For this review, take the finished solid that the model builds, in its own axes (mm). A direction names the side the tool comes from. Coordinates: 2 decimals unless noted, no trailing zeros. Loops run counter-clockwise (first coordinate to the right, second up) from the corner with the lowest first, then second, coordinate; pieces in that order, holes last.
1. Machinability: for faces 1 (the face through (32, 24, -11)), 2 (the face through (35.5, 16, -61)), 3 (the face through (62.479, 6.534, -25.903)), 4 (the face through (56.8, 20, -68)), 5 (the face through (27, 4, -1)), which of the approach directions +Z, -Z, +X, -X, +Y, -Y give a long, thin tool a straight path to every point of the face, cutting with its end or side? Answer none if there is none.
2. Mouldability with a two-part tool opening along Z and no side actions: class faces 6 (the face through (28.5, 16, -61)), 7 (the face through (32.149, 17.162, -90.403)), 8 (the face through (59.45, 22, -34)), 9 (the face through (32, 0, -82)) as pulls with the +Z half, pulls with the -Z half, needs draft (parallel to the pull), parting line crosses it, or undercut.
3. Take a section at A-A, the plane z = -53. State the section outline as (x, y) points.
4. Take a section at D-D, the plane z = -13.5. State the section outline as (x, y) points.
5. Take a section at C-C, the plane y = 2.25. State the section outline as (x, z) points, then the cut area to 3 significant figures.
6. To check wall thickness, follow probe 1 along Z at (x, y) = (19.5, 16.8); probe 2 along Z at (x, y) = (44.5, 15.5); probe 3 along X at (y, z) = (11, -19). State the ranges of each line that lie inside material, in increasing order.
7. Clearance check with flat-ended pins moving along their axes: P1, Ø1.1, axis at x = 8.5, z = -69.5, coming from the -Y side; P2, Ø2.5, axis at y = 5, z = -1.5, coming from the +X side; P3, Ø3, axis at x = 43, z = -59, coming from the +Y side. State where each tip first meets the part, or that it passes through.
8. Take a section at B-B, the plane x = 44.5. State the section outline as (y, z) points.
```python
from build123d import *

# Parameters (mm, degrees)
SKETCH1_W           = 64
SKETCH1_H           = 84.5
BOSS_EXTRUDE1_DEPTH = 27
FILLET1_R           = 5
SKETCH2_W           = 42.4
SKETCH2_H           = 61.5
CUT_EXTRUDE1_DEPTH  = 9.4
SKETCH3_W           = 3.6
SKETCH3_H           = 5.4
CUT_EXTRUDE2_DEPTH  = 61.5
SKETCH4_W           = 7
SKETCH4_H           = 4.8
CUT_EXTRUDE3_DEPTH  = 61.5
SKETCH5_W           = 58
SKETCH5_H           = 78.5
CUT_EXTRUDE4_DEPTH  = 14.6
FILLET2_R           = 5
CUT_EXTRUDE5_START  = -9.4
CUT_EXTRUDE5_DEPTH  = 9.4
SKETCH7_W           = 10
SKETCH7_H           = 10
CUT_EXTRUDE6_DEPTH  = 10
FILLET3_SIZE        = 1
SKETCH8_W           = 6.25
SKETCH8_H           = 13.5
CUT_EXTRUDE8_DEPTH  = 9.4
CUT_EXTRUDE9_DEPTH  = 10
SKETCH10_W          = 6.25
SKETCH10_H          = 9
CUT_EXTRUDE10_DEPTH = 9.4
SKETCH11_W          = 7
SKETCH11_H          = 1
SKETCH11_W_2        = 29.4
CUT_EXTRUDE11_DEPTH = 9.4
SKETCH12_W          = 29.4
SKETCH12_H          = 7.5
BOSS_EXTRUDE2_DEPTH = 3
SKETCH13_W          = 0.75
SKETCH13_H          = 27.9
CUT_EXTRUDE12_DEPTH = 3
SKETCH15_R          = 7.369867451
SKETCH15_R_2        = 7.5
CUT_EXTRUDE13_DEPTH = 3
BOSS_EXTRUDE3_DEPTH = 64
BOSS_EXTRUDE4_DEPTH = 27
SKETCH18_W          = 49.6
SKETCH18_H          = 7.565133063
CUT_EXTRUDE16_DEPTH = 5.4
SKETCH19_W          = 42.4
SKETCH19_H          = 4
CUT_EXTRUDE17_DEPTH = 5.4
CUT_EXTRUDE18_DEPTH = 3
SKETCH21_R          = 2
CUT_EXTRUDE19_DEPTH = 10


with BuildPart() as part:
    # Sketch1 → Boss-Extrude1 (new body)
    with BuildSketch(Plane(origin=(0, 0, 0), x_dir=(1, 0, 0), z_dir=(0, 1, 0))):
        with Locations((32, 42.25)):
            Rectangle(SKETCH1_W, SKETCH1_H)
    extrude(amount=BOSS_EXTRUDE1_DEPTH)

    # Fillet1
    fillet1_edges = [part.edges().sort_by_distance(p)[0] for p in [
        (0, 13.5, -84.5),
        (64, 13.5, -84.5),
        (64, 13.5, 0),
        (0, 13.5, 0),
    ]]
    fillet(fillet1_edges, radius=FILLET1_R)

    # Sketch2 → Cut-Extrude1 (cut)
    with BuildSketch(Plane(origin=(0, 27, 0), x_dir=(1, 0, 0), z_dir=(0, 1, 0))):
        with Locations((32, 53.75)):
            Rectangle(SKETCH2_W, SKETCH2_H)
    extrude(amount=-CUT_EXTRUDE1_DEPTH, mode=Mode.SUBTRACT)

    # Sketch3 → Cut-Extrude2 (cut)
    with BuildSketch(Plane(origin=(0, 0, -84.5), x_dir=(-1, 0, 0), z_dir=(0, 0, -1))):
        with Locations((-55, 20.3)):
            Rectangle(SKETCH3_W, SKETCH3_H)
        with Locations((-9, 20.3)):
            Rectangle(SKETCH3_W, SKETCH3_H)
    extrude(amount=-CUT_EXTRUDE2_DEPTH, mode=Mode.SUBTRACT)

    # Sketch4 → Cut-Extrude3 (cut)
    with BuildSketch(Plane(origin=(0, 17.6, 0), x_dir=(1, 0, 0), z_dir=(0, 1, 0))):
        Polygon((17.3, 23), (46.7, 23), (46.7, 49.4), (35.5, 49.4), (28.5, 49.4), (17.3, 49.4), align=None)
        with Locations((32, 51.8)):
            Rectangle(SKETCH4_W, SKETCH4_H)
    extrude(amount=-CUT_EXTRUDE3_DEPTH, mode=Mode.SUBTRACT)

    # Sketch5 → Cut-Extrude4 (cut)
    with BuildSketch(Plane.XZ):
        with Locations((32, -42.25)):
            Rectangle(SKETCH5_W, SKETCH5_H)
        Polygon((28.5, -54.2), (28.5, -49.4), (17.3, -49.4), (17.3, -23), (46.7, -23), (46.7, -49.4), (35.5, -49.4), (35.5, -54.2), align=None, mode=Mode.SUBTRACT)
    extrude(amount=-CUT_EXTRUDE4_DEPTH, mode=Mode.SUBTRACT)

    # Fillet2
    fillet2_edges = [part.edges().sort_by_distance(p)[0] for p in [
        (61, 7.3, -3),
        (61, 7.3, -81.5),
        (3, 7.3, -81.5),
        (3, 7.3, -3),
    ]]
    fillet(fillet2_edges, radius=FILLET2_R)

    # Sketch6 → Cut-Extrude5 (cut)
    with BuildSketch(Plane.XZ.offset(-14.6).offset(CUT_EXTRUDE5_START)):
        with BuildLine():
            Line((8, -3), (56, -3))
            ThreePointArc((56, -3), (59.535533906, -4.464466094), (61, -8))
            Line((61, -8), (61, -20))
            Line((61, -20), (56, -20))
            Line((56, -20), (8, -20))
            Line((8, -20), (3, -20))
            Line((3, -20), (3, -8))
            ThreePointArc((3, -8), (4.464466094, -4.464466094), (8, -3))
        make_face()
    extrude(amount=CUT_EXTRUDE5_DEPTH, mode=Mode.SUBTRACT)

    # Sketch7 → Cut-Extrude6 (cut)
    with BuildSketch(Plane.XY):
        with Locations((32, 5)):
            Rectangle(SKETCH7_W, SKETCH7_H)
    extrude(amount=-CUT_EXTRUDE6_DEPTH, mode=Mode.SUBTRACT)

    # Fillet3
    # a fillet whose section is not a circle: 1 mm, written as the material it adds along each edge
    with BuildSketch(Plane(origin=(37, 10, 0), x_dir=(0, -1, 0), z_dir=(0, 0, -1))) as fillet3_piece_1:
        with BuildLine():
            add(Edge.make_bspline([(FILLET3_SIZE, 0), (FILLET3_SIZE * 0.831801948466, 0), (FILLET3_SIZE * 0.663603896932, 0), (FILLET3_SIZE * 0.292893218813, FILLET3_SIZE * 0.0716919198361), (FILLET3_SIZE * 0.0716919198361, FILLET3_SIZE * 0.292893218813), (0, FILLET3_SIZE * 0.663603896932), (0, FILLET3_SIZE * 0.831801948466), (0, FILLET3_SIZE)], knots=[0, 0, 0, 0, 0, 0, 0.5, 0.5, 1, 1, 1, 1, 1, 1], degree=5))
            Line((0, FILLET3_SIZE), (0, 0))
            Line((0, 0), (FILLET3_SIZE, 0))
        make_face()
    extrude(amount=3)
    with BuildSketch(Plane(origin=(27, 10, 0), x_dir=(0, -1, 0), z_dir=(0, 0, -1))) as fillet3_piece_2:
        with BuildLine():
            add(Edge.make_bspline([(FILLET3_SIZE, 0), (FILLET3_SIZE * 0.831801948466, 0), (FILLET3_SIZE * 0.663603896932, 0), (FILLET3_SIZE * 0.292893218813, -FILLET3_SIZE * 0.0716919198361), (FILLET3_SIZE * 0.0716919198361, -FILLET3_SIZE * 0.292893218813), (0, -FILLET3_SIZE * 0.663603896932), (0, -FILLET3_SIZE * 0.831801948466), (0, -FILLET3_SIZE)], knots=[0, 0, 0, 0, 0, 0, 0.5, 0.5, 1, 1, 1, 1, 1, 1], degree=5))
            Line((0, -FILLET3_SIZE), (0, 0))
            Line((0, 0), (FILLET3_SIZE, 0))
        make_face()
    extrude(amount=3)

    # Sketch8 → Cut-Extrude8 (cut)
    with BuildSketch(Plane(origin=(0, 27, 0), x_dir=(1, 0, 0), z_dir=(0, 1, 0))):
        with Locations((7.675, 29.75)):
            Rectangle(SKETCH8_W, SKETCH8_H)
        with Locations((56.325, 29.75)):
            Rectangle(SKETCH8_W, SKETCH8_H)
    extrude(amount=-CUT_EXTRUDE8_DEPTH, mode=Mode.SUBTRACT)

    # Sketch9 → Cut-Extrude9 (cut)
    with BuildSketch(Plane(origin=(0, 17.6, 0), x_dir=(1, 0, 0), z_dir=(0, 1, 0))):
        Polygon((17.3, 49.4), (17.3, 57.4), (28.5, 57.4), (28.5, 62.2), (35.5, 62.2), (35.5, 57.4), (46.7, 57.4), (46.7, 49.4), align=None)
    extrude(amount=-CUT_EXTRUDE9_DEPTH, mode=Mode.SUBTRACT)

    # Sketch10 → Cut-Extrude10 (cut)
    with BuildSketch(Plane(origin=(0, 27, 0), x_dir=(1, 0, 0), z_dir=(0, 1, 0))):
        with Locations((7.675, 41)):
            Rectangle(SKETCH10_W, SKETCH10_H)
        with Locations((56.325, 41)):
            Rectangle(SKETCH10_W, SKETCH10_H)
    extrude(amount=-CUT_EXTRUDE10_DEPTH, mode=Mode.SUBTRACT)

    # Sketch11 → Cut-Extrude11 (cut)
    with BuildSketch(Plane(origin=(0, 17.6, 0), x_dir=(1, 0, 0), z_dir=(0, 1, 0))):
        with Locations((32, 62.7)):
            Rectangle(SKETCH11_W, SKETCH11_H)
        with Locations((32, 57.9)):
            Rectangle(SKETCH11_W_2, SKETCH11_H)
    extrude(amount=-CUT_EXTRUDE11_DEPTH, mode=Mode.SUBTRACT)

    # Sketch12 → Boss-Extrude2 (add)
    with BuildSketch(Plane.XZ.offset(-14.6)):
        with Locations((32, -26.75)):
            Rectangle(SKETCH12_W, SKETCH12_H)
    extrude(amount=-BOSS_EXTRUDE2_DEPTH)

    # Sketch13 → Cut-Extrude12 (cut)
    with BuildSketch(Plane(origin=(0, 17.6, 0), x_dir=(1, 0, 0), z_dir=(0, 1, 0))):
        with Locations((16.925, 44.45)):
            Rectangle(SKETCH13_W, SKETCH13_H)
        with Locations((47.075, 44.45)):
            Rectangle(SKETCH13_W, SKETCH13_H)
    extrude(amount=-CUT_EXTRUDE12_DEPTH, mode=Mode.SUBTRACT)

    # Sketch15 → Cut-Extrude13 (cut)
    with BuildSketch(Plane.XZ.offset(-14.6)):
        with Locations((44.5, -32.5)):
            Circle(SKETCH15_R)
        with Locations((19.5, -32.5)):
            Circle(SKETCH15_R_2)
    extrude(amount=-CUT_EXTRUDE13_DEPTH, mode=Mode.SUBTRACT)

    # Sketch16 → Boss-Extrude3 (add)
    with BuildSketch(Plane(origin=(64, 0, 0), x_dir=(0, 0, -1), z_dir=(1, 0, 0))):
        Polygon((84.5, 27), (84.5, 17), (84.5, 0), (90.5, 0), (90.5, 17), align=None)
    extrude(amount=-BOSS_EXTRUDE3_DEPTH)

    # Sketch17 → Boss-Extrude4 (add)
    with BuildSketch(Plane(origin=(0, 27, 0), x_dir=(1, 0, 0), z_dir=(0, 1, 0))):
        Polygon((64, 84.5), (64, 79.5), (59, 84.5), align=None)
        Polygon((0, 79.5), (5, 84.5), (0, 84.5), align=None)
    extrude(amount=-BOSS_EXTRUDE4_DEPTH)

    # Sketch18 → Cut-Extrude16 (cut)
    with BuildSketch(Plane(origin=(0, 17.6, 0), x_dir=(1, 0, 0), z_dir=(0, 1, 0))):
        with Locations((32, 88.282566532)):
            Rectangle(SKETCH18_W, SKETCH18_H)
    extrude(amount=CUT_EXTRUDE16_DEPTH, mode=Mode.SUBTRACT)

    # Sketch19 → Cut-Extrude17 (cut)
    with BuildSketch(Plane.XY.offset(-84.5)):
        with Locations((32, 25)):
            Rectangle(SKETCH19_W, SKETCH19_H)
    extrude(amount=-CUT_EXTRUDE17_DEPTH, mode=Mode.SUBTRACT)

    # Sketch20 → Cut-Extrude18 (cut)
    with BuildSketch(Plane(origin=(0, 17.6, 0), x_dir=(1, 0, 0), z_dir=(0, 1, 0))):
        Polygon((10.8, 84.5), (10.8, 87.8), (53.2, 87.8), (53.2, 84.5), (53.2, 82.5), (10.8, 82.5), align=None)
    extrude(amount=-CUT_EXTRUDE18_DEPTH, mode=Mode.SUBTRACT)

    # Sketch21 → Cut-Extrude19 (cut)
    with BuildSketch(Plane.ZY.offset(-61)):
        with Locations((-62.75, 7.3)):
            Circle(SKETCH21_R)
        with Locations((-27.75, 7.3)):
            Circle(SKETCH21_R)
    extrude(amount=-CUT_EXTRUDE19_DEPTH, mode=Mode.SUBTRACT)


solid = part.part
```
Results list:
1. face 1: -Y
1. face 2: +Y, -Y
1. face 3: +X
1. face 4: -Z
1. face 5: +Z, -Y
2. face 6: undercut
2. face 7: pulls with the -Z half
2. face 8: undercut
2. face 9: needs draft
3. outline: (0, 0) - (3, 0) - (3, 14.6) - (16.55, 14.6) - (16.55, 17.6) - (7.2, 17.6) - (7.2, 23) - (10.8, 23) - (10.8, 27) - (0, 27) - close; (47.45, 14.6) - (61, 14.6) - (61, 0) - (64, 0) - (64, 27) - (53.2, 27) - (53.2, 23) - (56.8, 23) - (56.8, 17.6) - (47.45, 17.6) - close
4. outline: (0, 0) - (3, 0) - (3, 24) - (61, 24) - (61, 0) - (64, 0) - (64, 27) - (0, 27) - close
5. outline: (0, -90.5) - (64, -90.5) - (64, -5) arc R5 ccw to (59, 0) - (37, 0) - (37, -3) - (56, -3) arc R5 cw to (61, -8) - (61, -76.5) arc R5 cw to (56, -81.5) - (8, -81.5) arc R5 cw to (3, -76.5) - (3, -8) arc R5 cw to (8, -3) - (27, -3) - (27, 0) - (5, 0) arc R5 ccw to (0, -5) - close
5. area: 1,220 mm2
6. probe 1: z = -90.5 to -87.8, -82.5 to -58.4, -25 to -20, -3 to 0
6. probe 2: z = -90.5 to -87.8, -82.5 to -58.4, -25.13 to -20, -3 to 0
6. probe 3: x = 0 to 3, 61 to 64
7. P1: stops at y = 14.6
7. P2: stops at x = 63.47
7. P3: stops at y = 17.6
8. outline: (0, -90.5) - (17, -90.5) - (17.6, -90.14) - (17.6, -87.8) - (14.6, -87.8) - (14.6, -82.5) - (17.6, -82.5) - (17.6, -58.4) - (14.6, -58.4) - (14.6, -81.5) - (0, -81.5) - close; (0, -3) - (24, -3) - (24, -20) - (14.6, -20) - (14.6, -25.13) - (17.6, -25.13) - (17.6, -23) - (27, -23) - (27, 0) - (0, 0) - close
